Check sheet for the modelled part. Datum: model origin and axes. Units: mm. A direction names the side the tool comes from. Give positions to 0.01 mm unless a question says otherwise; leave off trailing zeros. Write each loop counter-clockwise with the first axis right and the second up, starting at its lowest first coordinate (ties: lowest second). Pieces come first, ordered by that corner, then holes. Notation, with made-up numbers: (-13, 62.5) -> (23, 62.5) arc R27 cw to (23, 88.5) -> close; hole circle Ø11 at (64, 38). An arc over 180 degrees is marked (long way). Return JSON: item names as keys, results as strings.
from build123d import *

# Parameters (mm, degrees)
SKETCH_1_W      = 33
SKETCH_1_H      = 16
EXTRUDE_1_DEPTH = 2
EXTRUDE_2_DEPTH = 5.5
SKETCH_3_W      = 29
SKETCH_3_H      = 12
EXTRUDE_3_DEPTH = 13


with BuildPart() as part:
    # 草图1 → 凸台-拉伸1 (new body)
    with BuildSketch(Plane(origin=(0, 0, 0), x_dir=(1, 0, 0), z_dir=(0, 1, 0))):
        Rectangle(SKETCH_1_W, SKETCH_1_H)
    extrude(amount=EXTRUDE_1_DEPTH)

    # 草图2 → 凸台-拉伸2 (add, symmetric)
    with BuildSketch(Plane.XY):
        with BuildLine():
            ThreePointArc((-14.5, 2), (-1.99286503, 3.990553371), (9.496887626, 9.317495439))
            Line((9.496887626, 9.317495439), (14.5, 2))
            Line((14.5, 2), (-14.5, 2))
        make_face()
    extrude(amount=EXTRUDE_2_DEPTH, both=True)

    # 草图3 → 凸台-拉伸3 (add)
    with BuildSketch(Plane(origin=(0, 0, 0), x_dir=(1, 0, 0), z_dir=(0, 1, 0))):
        Rectangle(SKETCH_3_W, SKETCH_3_H)
    extrude(amount=-EXTRUDE_3_DEPTH)


solid = part.part
(1) Set-up check for faces 1 (the flat face through (14.5, -6, 0)), 2 (the flat face through (-1, 2, 6)), 3 (the flat face through (0, -6, -6)), 4 (the flat face through (0, -6, 6)), 5 (the flat face through (-14.5, -6, 0)): record each of +Z, -Z, +X, -X, +Y, -Y from which the full face is reachable in a straight line by a thin tool's end or side.
Reply:
{"face 1": "+Z, -Z, +X, -Y", "face 2": "+Y", "face 3": "-Z, +X, -X, -Y", "face 4": "+Z, +X, -X, -Y", "face 5": "+Z, -Z, -X, -Y"}
(2) Thickness scan on L1, parallel to Z at x = -0.5, y = -7.25; L2, parallel to Y at x = 13.5, z = 6.25; L3, parallel to X at y = -8.75, z = 5.5. Record the ranges inside material, lowest first.
Reply:
{"L1": "-6 to 6", "L2": "0 to 2", "L3": "-14.5 to 14.5"}
(3) Depth check by flat-ended pin: pin 1 Ø8 at (x, y) = (13, -6.5) entering from +Z; pin 2 Ø4 at (x, z) = (-0.5, -1.5) entering from +Y; pin 3 Ø5 at (x, z) = (-2, 6) entering from +Y. Enter the tip coordinate at first touch or a pass-through.
Reply:
{"pin 1": "z = 6", "pin 2": "y = 5.21", "pin 3": "y = 4.81"}
(4) Cross-section at A-A on z = -2.5. Enter the section's corners in (x, y).
Reply:
{"outline": "(-16.5, 0) -> (-14.5, 0) -> (-14.5, -13) -> (14.5, -13) -> (14.5, 0) -> (16.5, 0) -> (16.5, 2) -> (14.5, 2) -> (9.5, 9.32) arc R45.98 cw to (-14.5, 2) -> (-16.5, 2) -> close"}
(5) Cross-section at C-C on y = -5.75. Enter the section's corners in (x, z), then the cut area to 3 significant figures.
Reply:
{"outline": "(-14.5, -6) -> (14.5, -6) -> (14.5, 6) -> (-14.5, 6) -> close", "area": "348 mm^2"}
(6) Cross-section at D-D on x = 3.5. Enter the section's corners in (y, z).
Reply:
{"outline": "(-13, -6) -> (0, -6) -> (0, -8) -> (2, -8) -> (2, -5.5) -> (6.06, -5.5) -> (6.06, 5.5) -> (2, 5.5) -> (2, 8) -> (0, 8) -> (0, 6) -> (-13, 6) -> close"}
